Part model, mm, in its own coordinate system. Round coordinates to 2 decimals unless told otherwise and drop trailing zeros. Write each loop counter-clockwise with the first axis right and the second up, starting at its lowest first coordinate (ties: lowest second). Pieces come first, ordered by that corner, then holes.
1) Saw through at A-A on x = 8.89. Write the cut outline in (y, z).
2) Saw through at D-D on x = 3. Write the cut outline in (y, z), and give its area (3 significant figures).
3) Saw through at B-B on y = 1. Count the separate pieces of the cut face and the enclosed holes in it, and give its area (3 significant figures).
4) Flat gauge pin, fed straight in: pin 1 (0.9 mm diameter, centred on x = 11.43, z = -2.54, fed in from +Y). Where does the tip first touch, or does it go through?
5) Drill centre lines: L1, parallel to Z at x = 13.97, y = 1.05; L2, parallel to Z at x = 17.78, y = 0.9; L3, parallel to X at y = 0.45, z = -18.25. Where is each one in solid material? Low to high.
6) Saw through at C-C on z = -17.5. Write the cut outline in (x, y), and give its area (3 significant figures).
Autodesk Inventor part; units mm, degrees
ref_plane "YZ Plane" through (0, 0, 0) normal (1, 0, 0) x (0, 1, 0)
ref_plane "XZ Plane" through (0, 0, 0) normal (0, 1, 0) x (-1, 0, 0)
ref_plane "XY Plane" through (0, 0, 0) normal (0, 0, 1) x (1, 0, 0)
sketch "Sketch1" plane through (0, 0, 0) normal (0, 1, 0) x (-1, 0, 0)
  line L0 (-2.54, 0) -> (-17.78, 0)
  line L1 (-20.32, -2.54) -> (-20.32, -17.78)
  line L2 (-17.78, -20.32) -> (-2.54, -20.32)
  line L3 (0, -17.78) -> (0, -2.54)
  arc A0 (-2.54, -20.32) -> (0, -17.78) centre (-2.54, -17.78) ccw
  arc A1 (-20.32, -17.78) -> (-17.78, -20.32) centre (-17.78, -17.78) ccw
  arc A2 (-17.78, 0) -> (-20.32, -2.54) centre (-17.78, -2.54) ccw
  arc A3 (0, -2.54) -> (-2.54, 0) centre (-2.54, -2.54) ccw
  circle A4 centre (-2.54, -17.78) radius 1.27
  circle A5 centre (-17.78, -17.78) radius 1.27
  line L4 (0, -2.54) -> (-20.32, -2.54) construction
  circle A6 centre (-1.27, -2.54) radius 0.508
  circle A7 centre (-3.81, -2.54) radius 0.508
  circle A8 centre (-6.35, -2.54) radius 0.508
  circle A9 centre (-8.89, -2.54) radius 0.508
  circle A10 centre (-11.43, -2.54) radius 0.508
  circle A11 centre (-13.97, -2.54) radius 0.508
  circle A12 centre (-16.51, -2.54) radius 0.508
  circle A13 centre (-19.05, -2.54) radius 0.508
  point P0 (0, 0)
  point P1 (-20.32, -20.32)
  point P2 (-20.32, 0)
  point P3 (0, -20.32)
  dimension "d0" = 20.32
  dimension "d1" = 20.32
  dimension "d2" = 2.54
  dimension "d3" = 2.54
  dimension "d6" = 2.54
  dimension "d11" = 1.27
  dimension "d12" = 1.27
  dimension "d13" = 1.016
  dimension "d16" = 2.54
extrude "Extrusion1" add sketch "Sketch1" along normal blind 1.6
properties part number "LIS3DH footprint"
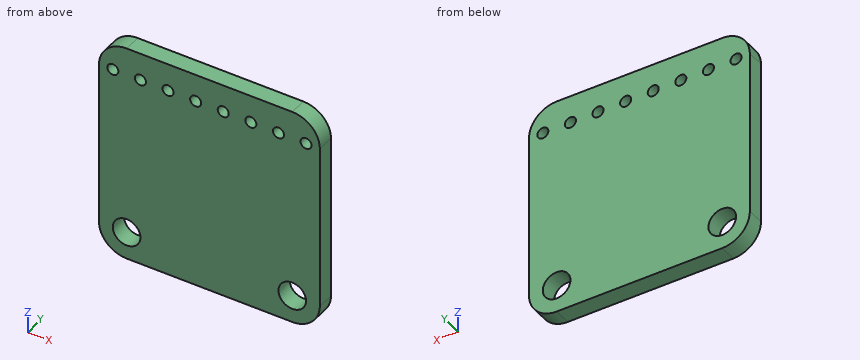
Completed:
1. outline: (0, -20.32) - (1.6, -20.32) - (1.6, -3.05) - (0, -3.05) - close; (0, -2.03) - (1.6, -2.03) - (1.6, 0) - (0, 0) - close
2. outline: (0, -20.32) - (1.6, -20.32) - (1.6, -18.96) - (0, -18.96) - close; (0, -16.6) - (1.6, -16.6) - (1.6, 0) - (0, 0) - close
2. area: 28.7 mm2
3. separate pieces: 1
3. enclosed holes: 10
3. area: 391 mm2
4. pin 1: passes through
5. L1: z = -20.32 to -3.05, -2.03 to 0
5. L2: z = -20.32 to -19.05, -16.51 to 0
5. L3: x = 0.04 to 1.36, 3.72 to 16.6, 18.96 to 20.28
6. outline: (0, 0) - (1.3, 0) - (1.3, 1.6) - (0, 1.6) - close; (3.78, 0) - (16.54, 0) - (16.54, 1.6) - (3.78, 1.6) - close; (19.02, 0) - (20.32, 0) - (20.32, 1.6) - (19.02, 1.6) - close
6. area: 24.6 mm2
